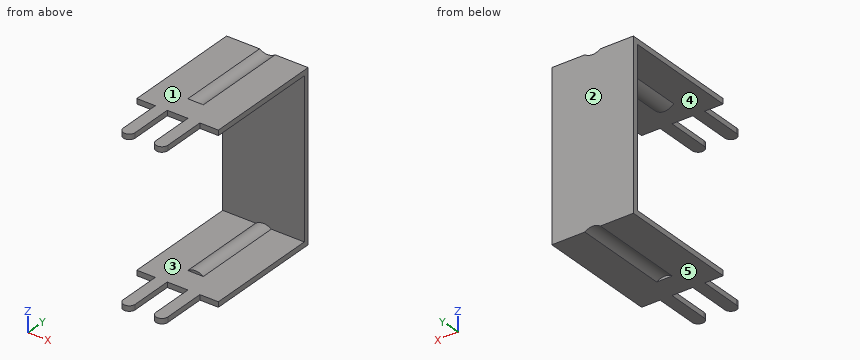
Autodesk Inventor part; units mm, degrees
ref_plane "bracket_to_switch_XY" through (0, 11.303, 0) normal (0, 1, 0) x (1, 0, 0)
ref_plane "bracket_to_switch_YZ" through (0, 11.303, 0) normal (1, 0, 0) x (0, 0, -1)
ref_plane "bracket_to_switch_ZX" through (0, 11.303, 0) normal (0, 0, -1) x (0, 1, 0)
sketch "Sketch_1" plane through (0, 0, 0) normal (1, 0, 0) x (0, 1, 0)
  line L0 (-4.8006, 8.1534) -> (-4.8006, 7.6454)
  line L1 (-4.8006, 7.6454) -> (11.303, 7.6454)
  line L2 (11.303, 7.6454) -> (11.303, -7.6454)
  line L3 (11.303, -7.6454) -> (-4.8006, -7.6454)
  line L4 (-4.8006, -7.6454) -> (-4.8006, -8.1534)
  line L5 (-4.8006, -8.1534) -> (11.811, -8.1534)
  line L6 (11.811, -8.1534) -> (11.811, 8.1534)
  line L7 (11.811, 8.1534) -> (-4.8006, 8.1534)
extrude "Extrusion1" add sketch "Sketch_1" along normal mid plane 8.001
sketch "Sketch_2" plane through (0, 0, 0) normal (0, 0, 1) x (1, 0, 0)
  line L0 (-4.0005, 0) -> (-4.0005, -4.953)
  line L1 (-4.0005, -4.953) -> (4.0005, -4.953)
  line L2 (4.0005, -4.953) -> (4.0005, 0)
  line L3 (4.0005, 0) -> (2.1844, 0)
  line L4 (2.1844, 0) -> (2.1844, -4.2164)
  arc A0 (1.016, -4.2164) -> (2.1844, -4.2164) centre (1.6002, -4.2164) ccw
  line L5 (1.016, -4.2164) -> (1.016, 0)
  line L6 (1.016, 0) -> (-1.016, 0)
  line L7 (-1.016, 0) -> (-1.016, -4.2164)
  arc A1 (-2.1844, -4.2164) -> (-1.016, -4.2164) centre (-1.6002, -4.2164) ccw
  line L8 (-2.1844, -4.2164) -> (-2.1844, 0)
  line L9 (-2.1844, 0) -> (-4.0005, 0)
extrude "Extrusion2" cut sketch "Sketch_2" along normal mid plane 16.3068
sketch "Sketch_3" plane through (0, 2.3622, 0) normal (0, 1, 0) x (1, 0, 0)
  arc A0 (-0.762, 7.6454) -> (0.762, 7.6454) centre (0, 8.6614) ccw
  line L0 (0.762, 7.6454) -> (-0.762, 7.6454)
extrude "Extrusion3" add sketch "Sketch_3" along normal blind 9.4488
sketch "Sketch_4" plane through (0, 2.3622, 0) normal (0, 1, 0) x (1, 0, 0)
  arc A0 (-1.27, 9.1694) -> (1.27, 9.1694) centre (0, 9.1694) ccw
  line L0 (1.27, 9.1694) -> (-1.27, 9.1694)
extrude "Extrusion4" cut sketch "Sketch_4" along normal blind 9.4488
sketch "Sketch_5" plane through (0, 2.3622, 0) normal (0, 1, 0) x (1, 0, 0)
  line L0 (-0.907, -7.6454) -> (0.907, -7.6454)
  arc A0 (0.907, -7.6454) -> (-0.907, -7.6454) centre (0, -8.5344) ccw
extrude "Extrusion5" add sketch "Sketch_5" along normal blind 9.4488
sketch "Sketch_6" plane through (0, 2.3622, 0) normal (0, 1, 0) x (1, 0, 0)
  line L0 (-1.27, -9.1694) -> (1.27, -9.1694)
  arc A0 (1.27, -9.1694) -> (-1.27, -9.1694) centre (0, -9.1694) ccw
extrude "Extrusion6" cut sketch "Sketch_6" along normal blind 9.4488
ref_plane "bracket_to_switch_XY" through (0, 11.303, 0) normal (0, 1, 0) x (1, 0, 0)
ref_plane "bracket_to_switch_YZ" through (0, 11.303, 0) normal (1, 0, 0) x (0, 0, -1)
ref_plane "bracket_to_switch_ZX" through (0, 11.303, 0) normal (0, 0, -1) x (0, 1, 0)
properties part number "BBRACKET13"
Could you check a few things on this model? Use its own coordinates, in mm. Face numbers are marked on the shaded views. A direction names the side the tool comes from. Coordinates: 2 decimals unless noted, no trailing zeros. Order: outer loops, then holes, each group sorted by start corner. A loop starts at its lowest first (then second) coordinate and runs counter-clockwise, first axis right, second up. Notation, with made-up numbers: (38, 51) - (73, 51) arc R20 cw to (73, 85) - close; hole circle Ø7 at (51.5, 54.5). An arc over 180 degrees is marked (long way). Answer in a Markdown table with one row per item. Add a question column.
(1) Will these pins go through, and if not, where does the flat tip stop? pin 1 (0.6 mm diameter, centred on x = 3.5, z = -8, fed in from -Y); pin 2 (4 mm diameter, centred on x = -1.5, z = 2.5, fed in from -Y); pin 3 (0.6 mm diameter, centred on y = -2, z = 8, fed in from -X); pin 4 (5 mm diameter, centred on y = 0.5, z = -4, fed in from -X).
(2) On a 3-axis mill with a long thin cutter (end or side, diameter ignored), from which of +Z, -Z, +X, -X, +Y, -Y can I reach the whole of each face in a straight line? I mean the marked faces 4 and 5. Say none if no direction works.
(3) If we mould it in two halves opening along Z, with no side actions, what happens to the marked faces 1, 2 and 3? For each: released by +Z, released by -Z, zero draft, split by the parting line, or undercut.
(4) If we section it at C-C, the plane x = -0.25: Please give me the cut outline in (y, z), then the cut area to 3 significant figures.
(5) If we section it at B-B, the plane y = -2.75: Please give me the cut outline in (x, z).
(6) I need wall thicknesses on L1, parallel to Z at x = -1, y = 3.25; L2, parallel to Y at x = 2, z = -3.75; L3, parallel to Z at x = 0.75, y = 5.75. Which ranges of each line are inside material? Lowest first, please.
(7) If we section it at A-A, the plane y = 4.75: Please give me the cut outline in (x, z).
(8) If we section it at D-D, the plane y = 1.5: Please give me the cut outline in (x, z).
Results are:
| question | item | result |
|---|---|---|
| 1 | pin 1 | stops at y = 0 |
| 1 | pin 2 | stops at y = 11.3 |
| 1 | pin 3 | stops at x = -2.18 |
| 1 | pin 4 | passes through |
| 2 | face 4 | -Y |
| 2 | face 5 | -Z, +X, -X, +Y, -Y |
| 3 | face 1 | released by +Z |
| 3 | face 2 | zero draft |
| 3 | face 3 | undercut |
| 4 | outline | (0, -8.15) - (2.36, -8.15) - (2.36, -7.92) - (11.81, -7.92) - (11.81, 7.92) - (2.36, 7.92) - (2.36, 8.15) - (0, 8.15) - (0, 7.65) - (2.36, 7.65) - (2.36, 7.29) - (11.3, 7.29) - (11.3, -7.42) - (2.36, -7.42) - (2.36, -7.65) - (0, -7.65) - close |
| 4 | area | 20.7 mm2 |
| 5 | outline | (-2.18, -8.15) - (-1.02, -8.15) - (-1.02, -7.65) - (-2.18, -7.65) - close; (-2.18, 7.65) - (-1.02, 7.65) - (-1.02, 8.15) - (-2.18, 8.15) - close; (1.02, -8.15) - (2.18, -8.15) - (2.18, -7.65) - (1.02, -7.65) - close; (1.02, 7.65) - (2.18, 7.65) - (2.18, 8.15) - (1.02, 8.15) - close |
| 6 | L1 | z = -8.15 to -7.65, 7.65 to 8.15 |
| 6 | L2 | y = 11.3 to 11.81 |
| 6 | L3 | z = -8.14 to -7.64, 7.51 to 8.14 |
| 7 | outline | (-4, -8.15) - (-0.76, -8.15) arc R1.27 cw to (0.76, -8.15) - (4, -8.15) - (4, -7.65) - (0.76, -7.65) arc R1.27 ccw to (-0.76, -7.65) - (-4, -7.65) - close; (-4, 7.65) - (-0.91, 7.65) arc R1.27 ccw to (0.91, 7.65) - (4, 7.65) - (4, 8.15) - (0.76, 8.15) arc R1.27 cw to (-0.76, 8.15) - (-4, 8.15) - close |
| 8 | outline | (-4, -8.15) - (4, -8.15) - (4, -7.65) - (-4, -7.65) - close; (-4, 7.65) - (4, 7.65) - (4, 8.15) - (-4, 8.15) - close |
